```python
from build123d import *

# Parameters (mm, degrees)
BOSS_EXTRUDE1_DEPTH     = 10.5
SKETCH2_W               = 10
SKETCH2_H               = 6
SKETCH2_W_2             = 0.8
SKETCH2_H_2             = 3
CUT_EXTRUDE1_DEPTH      = 10.5
M1_4X0_3_TAPPED_HOLE1_D = 1.1
SKETCH4_W               = 0.7
SKETCH4_H               = 1.8
BOSS_EXTRUDE2_DEPTH     = 0.5
FILLET1_R               = 0.5


with BuildPart() as part:
    # Sketch1 → Boss-Extrude1 (new, symmetric)
    with BuildSketch(Plane(origin=(0, 0, 0), x_dir=(0, 0, -1), z_dir=(1, 0, 0))):
        with BuildLine():
            Line((-0.5, 3.692330317), (-0.5, 5))
            Line((-0.5, 5), (0.5, 5))
            Line((0.5, 5), (0.5, 3.692330317))
            ThreePointArc((0.5, 3.692330317), (1.153256259, 4.206274607), (1.4, 5))
            ThreePointArc((1.4, 5), (-0.793725393, 6.153256259), (-0.5, 3.692330317))
        make_face()
        with BuildLine():
            Line((0.5, 5), (-0.5, 5))
            Line((-0.5, 5), (-0.5, 3.692330317))
            ThreePointArc((-0.5, 3.692330317), (0, 3.6), (0.5, 3.692330317))
            Line((0.5, 3.692330317), (0.5, 5))
        make_face()
        with BuildLine():
            ThreePointArc((0.5, 3.692330317), (0, 3.6), (-0.5, 3.692330317))
            Line((-0.5, 3.692330317), (-0.5, -5))
            Line((-0.5, -5), (0.5, -5))
            Line((0.5, -5), (0.5, 3.692330317))
        make_face()
    extrude(amount=BOSS_EXTRUDE1_DEPTH, both=True)

    # Sketch2 → Cut-Extrude1 (cut, symmetric)
    with BuildSketch(Plane.XY.offset(0.5)):
        with Locations((0, -2)):
            Rectangle(SKETCH2_W, SKETCH2_H)
        with Locations((-4.9, 4.9)):
            Rectangle(SKETCH2_W_2, SKETCH2_H_2)
        with BuildLine():
            Line((-6.5, 1.5), (-6.5, -2.5))
            ThreePointArc((-6.5, -2.5), (-8, -4), (-9.5, -2.5))
            Line((-9.5, -2.5), (-9.5, 1.5))
            ThreePointArc((-9.5, 1.5), (-8, 3), (-6.5, 1.5))
        make_face()
        with BuildLine():
            Line((6.5, 1.5), (6.5, -2.5))
            ThreePointArc((6.5, -2.5), (8, -4), (9.5, -2.5))
            Line((9.5, -2.5), (9.5, 1.5))
            ThreePointArc((9.5, 1.5), (8, 3), (6.5, 1.5))
        make_face()
        with Locations((4.9, 4.9)):
            Rectangle(SKETCH2_W_2, SKETCH2_H_2)
    extrude(amount=CUT_EXTRUDE1_DEPTH, both=True, mode=Mode.SUBTRACT)

    # M1.4x0.3 Tapped Hole1 (through all)
    with Locations(Plane(origin=(10.5, 5, 0), x_dir=(0, 0, 1), z_dir=(1, 0, 0))):
        with Locations((0, 0)):
            Hole(M1_4X0_3_TAPPED_HOLE1_D / 2)

    # Sketch4 → Boss-Extrude2 (add, symmetric)
    with BuildSketch(Plane.XY):
        with Locations((10.85, -3.207669683)):
            Rectangle(SKETCH4_W, SKETCH4_H)
    boss_extrude2 = extrude(amount=BOSS_EXTRUDE2_DEPTH, both=True)

    # Mirror1: Boss-Extrude2 across plane
    add(boss_extrude2.mirror(Plane(origin=(0, 0, 0), x_dir=(0, 0, 1), z_dir=(1, 0, 0))))

    # Fillet1
    fillet1_edges = [part.edges().sort_by_distance(p)[0] for p in [
        (-5, -5, 0),
        (-5, 1, 0),
        (5, 1, 0),
        (5, -5, 0),
    ]]
    fillet(fillet1_edges, radius=FILLET1_R)


solid = part.part
```
The listing builds one solid part. Answer for the finished solid, in the listing's coordinates (mm). A direction names the side the tool comes from. Coordinates: 2 decimals unless noted, no trailing zeros. Write each loop counter-clockwise with the first axis right and the second up, starting at its lowest first coordinate (ties: lowest second). Pieces come first, ordered by that corner, then holes. Notation, with made-up numbers: (-35, -1) - (-23, -1) arc R25 ccw to (-23, 19) - close; hole circle Ø9 at (15, 52.5). An arc over 180 degrees is marked (long way). Return JSON: item names as keys, results as strings. Group by question number.
1. Straight lines are drawn through the part: L1, parallel to X at y = 5.25, z = -0.6; L2, parallel to Z at x = 8.05, y = 5; L3, parallel to X at y = -2.75, z = 0. For each, find the intervals that lie inside material, in ascending order.
2. A cutting plane is placed at C-C, the plane y = 5. Determine the outline of the cut face in (x, z).
3. A cutting plane is placed at D-D, the plane z = 0. Give the number of separate pieces and of enclosed holes in the cut face, plus the area to 3 significant figures.
4. A cutting plane is placed at A-A, the plane x = 8. Determine the outline of the cut face in (y, z).
5. Determine the mould class of faces 1 (the flat face through (10.5, 3, 0)), 2 (the cylindrical face through (-7.936, 5.537, 0.119)), 3 (the flat face through (0.2, 1.2, -0.5)), 4 (the cylindrical face through (-0.063, 5.537, 0.119)) for opening direction Z: released by +Z, released by -Z, zero draft, split by the parting line, or undercut.
6. A cutting plane is placed at B-B, the plane y = -1. Determine the outline of the cut face in (x, z), plus the area to 3 significant figures.
7. Given pin 1 (1.4 mm diameter, centred on y = 4, z = 0.5, fed in from +X); pin 2 (1.5 mm diameter, centred on y = -0.5, z = 0.5, fed in from -X); pin 3 (1 mm diameter, centred on y = -4.5, z = 0, fed in from +X); pin 4 (2.5 mm diameter, centred on x = 0, y = 1.5, fed in from +Z), each flat-ended and moving along its own axis, determine where each tip first touches the part or whether it passes through.
8. Which of the six approach directions +Z, -Z, +X, -X, +Y, -Y give full straight-line access (tool end or side, diameter ignored) to faces 5 (the flat face through (10.5, -4.5, 0)), 6 (the flat face through (-9.5, -1, 0)), 7 (the flat face through (0.2, 1.3, 0.5)), 8 (the flat face through (-5.3, 5, -1))?
Ans:
{
 "1": {"L1": "-10.5 to -5.3, -4.5 to 4.5, 5.3 to 10.5", "L2": "-1.4 to -0.55, 0.55 to 1.4", "L3": "-11.2 to -9.48, -6.52 to -5, 5 to 6.52, 9.48 to 11.2"},
 "2": {"outline": "(-10.5, -1.4) - (-5.3, -1.4) - (-5.3, -0.55) - (-10.5, -0.55) - close; (-10.5, 0.55) - (-5.3, 0.55) - (-5.3, 1.4) - (-10.5, 1.4) - close; (-4.5, -1.4) - (4.5, -1.4) - (4.5, -0.55) - (-4.5, -0.55) - close; (-4.5, 0.55) - (4.5, 0.55) - (4.5, 1.4) - (-4.5, 1.4) - close; (5.3, -1.4) - (10.5, -1.4) - (10.5, -0.55) - (5.3, -0.55) - close; (5.3, 0.55) - (10.5, 0.55) - (10.5, 1.4) - (5.3, 1.4) - close"},
 "3": {"separate pieces": "4", "enclosed holes": "2", "area": "118 mm²"},
 "4": {"outline": "(-5, -0.5) - (-4, -0.5) - (-4, 0.5) - (-5, 0.5) - close; (3, -0.5) - (3.69, -0.5) arc R1.4 ccw (long way) to (3.69, 0.5) - (3, 0.5) - close; hole circle Ø1.1 at (5, 0)"},
 "5": {"face 1": "zero draft", "face 2": "undercut", "face 3": "released by -Z", "face 4": "undercut"},
 "6": {"outline": "(-10.5, -0.5) - (-9.5, -0.5) - (-9.5, 0.5) - (-10.5, 0.5) - close; (-6.5, -0.5) - (-5, -0.5) - (-5, 0.5) - (-6.5, 0.5) - close; (5, -0.5) - (6.5, -0.5) - (6.5, 0.5) - (5, 0.5) - close; (9.5, -0.5) - (10.5, -0.5) - (10.5, 0.5) - (9.5, 0.5) - close", "area": "5.00 mm²"},
 "7": {"pin 1": "x = 10.5", "pin 2": "x = -10.5", "pin 3": "x = 11.2", "pin 4": "z = 0.5"},
 "8": {"face 5": "+Z, -Z, +X, -Y", "face 6": "+Z, -Z", "face 7": "+Z, +X, -X, -Y", "face 8": "+Z, -Z, +Y"}
}
